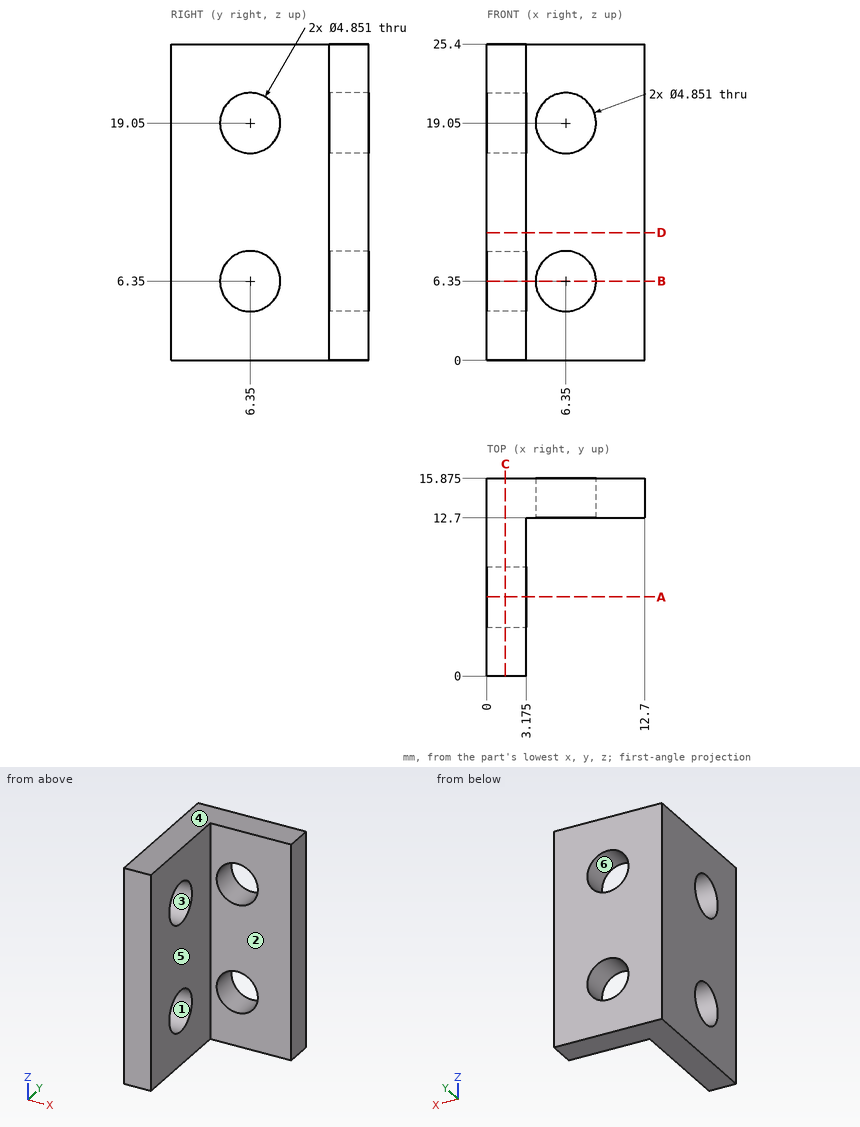
Study the drawing (mm; zero at the part's minimum x, y, z) and answer. A direction names the side the tool comes from. Coordinates: 2 decimals unless noted, no trailing zeros. Write each loop counter-clockwise with the first axis right and the second up, starting at its lowest first coordinate (ties: lowest second). Pieces come first, ordered by that corner, then holes. Notation, with made-up numbers: M 65.5,58 L 100.5,58 A17 cw 100.5,84 Z; hole C 53.5,-6.75 d9. An arc over 180 degrees is marked long. Use a Markdown table: item, result. Add a question column.
1. Section D-D (z = 10.25) is taken. Give the vertices of the cut face in (x, y) (1 decimal).
2. Section A-A (y = 6.35) is taken. Give the vertices of the cut face in (x, z) (1 decimal).
3. Straight lines are drawn through the part: line 1 along Z through (x, y) = (6.35, 14.45) (1 decimal); line 2 along Y through (x, z) = (1.2, 6.35) (1 decimal); line 3 along Z through (x, y) = (1.75, 4.5). For each, find the intervals that lie inside material, in ascending order. Write a range as [from, to].
4. Given P1, Ø7.5, axis at x = 8.5, z = 18, coming from the -Y side; P2, Ø2, axis at y = 3.5, z = 8, coming from the +X side (3 decimals), each flat-ended and moving along its own axis, determine where each tip first touches the part or whether it passes through.
5. Section C-C (x = 1.5) is taken. Count the separate pieces of the cut face and the enclosed holes in it, plus the area to 3 significant figures.
6. Which of the six approach directions +Z, -Z, +X, -X, +Y, -Y give full straight-line access (tool end or side, diameter ignored) to the marked faces 5 and 6?
7. For a pull along Y with two mould halves and no side action, classify the marked faces 1, 2, 3 and 4 as +Y half, -Y half, draft (parallel to the pull), parting line (faces both ways), or undercut.
8. Section B-B (z = 6.35) is taken. Give the vertices of the cut face in (x, y) (1 decimal).
Data:
| question | item | result |
|---|---|---|
| 1 | outline | M 0,0 L 3.2,0 L 3.2,12.7 L 12.7,12.7 L 12.7,15.9 L 0,15.9 Z |
| 2 | outline | M 0,0 L 3.2,0 L 3.2,3.9 L 0,3.9 Z; M 0,8.8 L 3.2,8.8 L 3.2,16.6 L 0,16.6 Z; M 0,21.5 L 3.2,21.5 L 3.2,25.4 L 0,25.4 Z |
| 3 | line 1 | z = [0, 3.9], [8.8, 16.6], [21.5, 25.4] |
| 3 | line 2 | y = [0, 3.9], [8.8, 15.9] |
| 3 | line 3 | z = [0, 4.78], [7.92, 17.48], [20.62, 25.4] |
| 4 | P1 | stops at y = 12.7 |
| 4 | P2 | stops at x = 3.175 |
| 5 | separate pieces | 1 |
| 5 | enclosed holes | 2 |
| 5 | area | 366 mm2 |
| 6 | face 5 | +Z, -Z, +X, -Y |
| 6 | face 6 | +Y, -Y |
| 7 | face 1 | undercut |
| 7 | face 2 | -Y half |
| 7 | face 3 | undercut |
| 7 | face 4 | draft |
| 8 | outline | M 0,0 L 3.2,0 L 3.2,3.9 L 0,3.9 Z; M 0,8.8 L 3.2,8.8 L 3.2,12.7 L 3.9,12.7 L 3.9,15.9 L 0,15.9 Z; M 8.8,12.7 L 12.7,12.7 L 12.7,15.9 L 8.8,15.9 Z |
